from build123d import *

# Parameters (mm, degrees)
BOSS_EXTRUDE1_DEPTH            = 29
SKETCH2_R                      = 2.6
SKETCH2_R_2                    = 1.55
BOSS_EXTRUDE3_DEPTH            = 5
CUT_EXTRUDE1_REACH             = 90.599
CUT_EXTRUDE1_DIRECTION_2_DEPTH = 89.598840586
CUT_EXTRUDE2_REACH             = 90.599
CUT_EXTRUDE2_DIRECTION_2_DEPTH = 89.598840586
FILLET1_R                      = 2
SKETCH6_R                      = 2.6
BOSS_EXTRUDE4_DEPTH            = 1


with BuildPart() as part:
    # Sketch1 → Boss-Extrude1 (new body)
    with BuildSketch(Plane(origin=(0, 0, 0), x_dir=(1, 0, 0), z_dir=(0, 1, 0))):
        Polygon((-13.5, 0), (0, 74.39897269), (13.5, 0), (14.483932895, 0.178538676), (0, 80), (-14.483932895, 0.178538676), align=None)
    extrude(amount=BOSS_EXTRUDE1_DEPTH)

    # Sketch2 → Boss-Extrude3 (add)
    # profile 1 of 8: a face of its own
    with BuildSketch(Plane(origin=(0, 0, 0), x_dir=(1, 0, 0), z_dir=(0, 1, 0))):
        with Locations((11.925707369, -0.285661882)):
            Circle(SKETCH2_R)
        with Locations(Location((11.925707369, -0.285661882, 0), (0, 0, 270))):
            Circle(SKETCH2_R_2, mode=Mode.SUBTRACT)
    # profile 2 of 8: a face of its own
    with BuildSketch(Plane(origin=(0, 0, 0), x_dir=(1, 0, 0), z_dir=(0, 1, 0))):
        with Locations((9.426165905, 13.489398644)):
            Circle(SKETCH2_R)
        with Locations(Location((9.426165905, 13.489398644, 0), (0, 0, 270))):
            Circle(SKETCH2_R_2, mode=Mode.SUBTRACT)
    # profile 3 of 8: a face of its own
    with BuildSketch(Plane(origin=(0, 0, 0), x_dir=(1, 0, 0), z_dir=(0, 1, 0))):
        with Locations((6.926624441, 27.264459169)):
            Circle(SKETCH2_R)
        with Locations(Location((6.926624441, 27.264459169, 0), (0, 0, 270))):
            Circle(SKETCH2_R_2, mode=Mode.SUBTRACT)
    # profile 4 of 8: a face of its own
    with BuildSketch(Plane(origin=(0, 0, 0), x_dir=(1, 0, 0), z_dir=(0, 1, 0))):
        with Locations((4.427082978, 41.039519694)):
            Circle(SKETCH2_R)
        with Locations(Location((4.427082978, 41.039519694, 0), (0, 0, 270))):
            Circle(SKETCH2_R_2, mode=Mode.SUBTRACT)
    # profile 5 of 8: a face of its own
    with BuildSketch(Plane(origin=(0, 0, 0), x_dir=(1, 0, 0), z_dir=(0, 1, 0))):
        with Locations((-11.925707369, -0.285661882)):
            Circle(SKETCH2_R)
        with Locations(Location((-11.925707369, -0.285661882, 0), (0, 0, 90))):
            Circle(SKETCH2_R_2, mode=Mode.SUBTRACT)
    # profile 6 of 8: a face of its own
    with BuildSketch(Plane(origin=(0, 0, 0), x_dir=(1, 0, 0), z_dir=(0, 1, 0))):
        with Locations((-9.426165905, 13.489398644)):
            Circle(SKETCH2_R)
        with Locations(Location((-9.426165905, 13.489398644, 0), (0, 0, 90))):
            Circle(SKETCH2_R_2, mode=Mode.SUBTRACT)
    # profile 7 of 8: a face of its own
    with BuildSketch(Plane(origin=(0, 0, 0), x_dir=(1, 0, 0), z_dir=(0, 1, 0))):
        with Locations((-6.926624441, 27.264459169)):
            Circle(SKETCH2_R)
        with Locations(Location((-6.926624441, 27.264459169, 0), (0, 0, 90))):
            Circle(SKETCH2_R_2, mode=Mode.SUBTRACT)
    # profile 8 of 8: a face of its own
    with BuildSketch(Plane(origin=(0, 0, 0), x_dir=(1, 0, 0), z_dir=(0, 1, 0))):
        with Locations((-4.427082978, 41.039519694)):
            Circle(SKETCH2_R)
        with Locations(Location((-4.427082978, 41.039519694, 0), (0, 0, 90))):
            Circle(SKETCH2_R_2, mode=Mode.SUBTRACT)
    boss_extrude3 = extrude(amount=BOSS_EXTRUDE3_DEPTH)

    # Cut-Extrude1: up to this face of the body (flat: up to its plane)
    cut_extrude1_end = Plane(part.part.faces().sort_by_distance((-6.66752213, 14.905805763, -37.654024776))[0])
    # Sketch4 → Cut-Extrude1 (cut, up to the picked face)
    with BuildSketch(Plane(origin=(0.430326794, 0, 2.371546029), x_dir=(0.9839328946538309, 0, -0.17853867597283662), z_dir=(0.17853867597283662, 0, 0.9839328946538309)), mode=Mode.PRIVATE) as cut_extrude1_sk1:
        Polygon((13.283094078, 5), (9.083094078, 5), (9.083094078, 1.475781549), align=None)
    cut_extrude1_tool1 = split(extrude(cut_extrude1_sk1.sketch, amount=-CUT_EXTRUDE1_REACH, mode=Mode.PRIVATE), bisect_by=cut_extrude1_end, keep=Keep.BOTH, mode=Mode.PRIVATE)
    cut_extrude1 = cut_extrude1_tool1.solids().sort_by(Axis((10.744988, 3.825261, 0.499908), (-0.17853867597283662, 0, -0.9839328946538309)))[0]
    add(cut_extrude1, mode=Mode.SUBTRACT)

    # Sketch4 → Cut-Extrude1 direction 2 (cut)
    with BuildSketch(Plane(origin=(0.430326794, 0, 2.371546029), x_dir=(0.9839328946538309, 0, -0.17853867597283662), z_dir=(0.17853867597283662, 0, 0.9839328946538309))):
        Polygon((13.283094078, 5), (9.083094078, 5), (9.083094078, 1.475781549), align=None)
    cut_extrude1_direction_2 = extrude(amount=CUT_EXTRUDE1_DIRECTION_2_DEPTH, mode=Mode.SUBTRACT)

    # Cut-Extrude2: up to this face of the body (flat: up to its plane)
    cut_extrude2_end = Plane(part.part.faces().sort_by_distance((6.66752213, 14.905805763, -37.654024776))[0])
    # Sketch5 → Cut-Extrude2 (cut, up to the picked face)
    with BuildSketch(Plane(origin=(-0.430326794, 0, 2.371546029), x_dir=(0.9839328946538308, 0, 0.17853867597283732), z_dir=(-0.17853867597283732, 0, 0.9839328946538308)), mode=Mode.PRIVATE) as cut_extrude2_sk1:
        Polygon((-9.083094078, 5), (-9.083094078, 1.475781549), (-13.283094078, 5), align=None)
    cut_extrude2_tool1 = split(extrude(cut_extrude2_sk1.sketch, amount=-CUT_EXTRUDE2_REACH, mode=Mode.PRIVATE), bisect_by=cut_extrude2_end, keep=Keep.BOTH, mode=Mode.PRIVATE)
    cut_extrude2 = cut_extrude2_tool1.solids().sort_by(Axis((-10.744988, 3.825261, 0.499908), (0.17853867597283732, 0, -0.9839328946538308)))[0]
    add(cut_extrude2, mode=Mode.SUBTRACT)

    # Sketch5 → Cut-Extrude2 direction 2 (cut)
    with BuildSketch(Plane(origin=(-0.430326794, 0, 2.371546029), x_dir=(0.9839328946538308, 0, 0.17853867597283732), z_dir=(-0.17853867597283732, 0, 0.9839328946538308))):
        Polygon((-9.083094078, 5), (-9.083094078, 1.475781549), (-13.283094078, 5), align=None)
    cut_extrude2_direction_2 = extrude(amount=CUT_EXTRUDE2_DIRECTION_2_DEPTH, mode=Mode.SUBTRACT)

    # Mirror2: Boss-Extrude3, Cut-Extrude1, Cut-Extrude1 direction 2, Cut-Extrude2, Cut-Extrude2 direction 2 across plane
    add(boss_extrude3.mirror(Plane.ZX.offset(14.5)))
    add(cut_extrude1.mirror(Plane.ZX.offset(14.5)), mode=Mode.SUBTRACT)
    add(cut_extrude1_direction_2.mirror(Plane.ZX.offset(14.5)), mode=Mode.SUBTRACT)
    add(cut_extrude2.mirror(Plane.ZX.offset(14.5)), mode=Mode.SUBTRACT)
    add(cut_extrude2_direction_2.mirror(Plane.ZX.offset(14.5)), mode=Mode.SUBTRACT)

    # Fillet1
    # the kernel refuses this fillet: 2 mm, written as the material it adds along each edge
    with BuildSketch(Plane(origin=(13.5, 5, 0), x_dir=(0, 1, 0), z_dir=(0.9839328946538308, 0, -0.17853867597283668))) as fillet1_piece_1_section:
        with BuildLine():
            CenterArc((FILLET1_R, FILLET1_R), FILLET1_R, 180, 90)
            Line((0, FILLET1_R), (0, 0))
            Line((0, 0), (FILLET1_R, 0))
        make_face()
    fillet1_piece_1 = extrude(amount=6, mode=Mode.PRIVATE)
    fillet1_piece_1 = fillet1_piece_1 & Plane(origin=(11.925707369, 5.699977743, 0.285661882), x_dir=(1, 0, 0), z_dir=(0, -1, 0)) * Cylinder(2.6, 20, mode=Mode.PRIVATE)
    add(fillet1_piece_1)
    with BuildSketch(Plane(origin=(13.5, 24, 0), x_dir=(0, -1, 0), z_dir=(0.9839328946538308, 0, -0.17853867597283668))) as fillet1_piece_2_section:
        with BuildLine():
            CenterArc((FILLET1_R, -FILLET1_R), FILLET1_R, 90, 90)
            Line((0, -FILLET1_R), (0, 0))
            Line((0, 0), (FILLET1_R, 0))
        make_face()
    fillet1_piece_2 = extrude(amount=6, mode=Mode.PRIVATE)
    fillet1_piece_2 = fillet1_piece_2 & Plane(origin=(11.925707369, 23.300022258, 0.285661882), x_dir=(1, 0, 0), z_dir=(0, 1, 0)) * Cylinder(2.6, 20, mode=Mode.PRIVATE)
    add(fillet1_piece_2)
    with BuildSketch(Plane(origin=(-19.403597368, 24, -1.071232056), x_dir=(0, -1, 0), z_dir=(0.9839328946538307, 0, 0.17853867597283735))) as fillet1_piece_3_section:
        with BuildLine():
            CenterArc((FILLET1_R, -FILLET1_R), FILLET1_R, 90, 90)
            Line((0, -FILLET1_R), (0, 0))
            Line((0, 0), (FILLET1_R, 0))
        make_face()
    fillet1_piece_3 = extrude(amount=6, mode=Mode.PRIVATE)
    fillet1_piece_3 = fillet1_piece_3 & Plane(origin=(-11.925707369, 23.777637105, 0.285661882), x_dir=(1, 0, 0), z_dir=(0, 1, 0)) * Cylinder(2.6, 21, mode=Mode.PRIVATE)
    add(fillet1_piece_3)
    with BuildSketch(Plane(origin=(-19.403597368, 5, -1.071232056), x_dir=(-0.17853867597283735, 0, 0.9839328946538307), z_dir=(0.9839328946538307, 0, 0.17853867597283735))) as fillet1_piece_4_section:
        with BuildLine():
            CenterArc((FILLET1_R, -FILLET1_R), FILLET1_R, 90, 90)
            Line((0, -FILLET1_R), (0, 0))
            Line((0, 0), (FILLET1_R, 0))
        make_face()
    fillet1_piece_4 = extrude(amount=6, mode=Mode.PRIVATE)
    fillet1_piece_4 = fillet1_piece_4 & Plane(origin=(-11.925707369, 5.222362792, 0.285661882), x_dir=(1, 0, 0), z_dir=(0, -1, 0)) * Cylinder(2.6, 21, mode=Mode.PRIVATE)
    add(fillet1_piece_4)

    # Sketch6 → Boss-Extrude4 (add)
    with BuildSketch(Plane.XZ):
        with Locations((4.427082978, -41.039519694)):
            Circle(SKETCH6_R)
        with Locations((-4.427082978, -41.039519694)):
            Circle(SKETCH6_R)
        with Locations((-6.926624441, -27.264459169)):
            Circle(SKETCH6_R)
        with Locations((11.925707369, 0.285661882)):
            Circle(SKETCH6_R)
        with Locations((6.926624441, -27.264459169)):
            Circle(SKETCH6_R)
        with Locations((9.426165905, -13.489398644)):
            Circle(SKETCH6_R)
        with Locations((-9.426165905, -13.489398644)):
            Circle(SKETCH6_R)
        with Locations((-11.925707369, 0.285661882)):
            Circle(SKETCH6_R)
    extrude(amount=-BOSS_EXTRUDE4_DEPTH)


solid = part.part
For this review, take the finished solid that the model builds, in its own axes (mm). A direction names the side the tool comes from. Round coordinates to 2 decimals unless told otherwise and drop trailing zeros. Write each loop counter-clockwise with the first axis right and the second up, starting at its lowest first coordinate (ties: lowest second). Pieces come first, ordered by that corner, then holes. Notation, with made-up numbers: (34.5, -27) - (39.5, -27) arc R23 ccw to (39.5, 5) - close; hole circle Ø6 at (25.25, 9.5). An arc over 180 degrees is marked (long way). Write item = value, one per line. Start each with the question number.
1. For faces 1 (the face through (-5.29, 26.57, -28.1)), 2 (the face through (5.964, 2.513, -41.241)), 3 (the face through (-7.026, 14.297, -35.681)), list the 3-axis set-ups (+Z, -Z, +X, -X, +Y, -Y) from which the entire face can be reached by the end or side of a thin tool; tool diameter is ignored.
2. Consider section B-B on y = 14.25. State the section outline as (x, z) points.
3. Consider section C-C on x = -1. State the section outline as (y, z) points.
4. Consider section A-A on z = -22. State the section outline as (x, y) points.
5. Wall thickness on L1, parallel to X at y = 1.5, z = -25; L2, parallel to X at y = 8.25, z = -2; L3, parallel to Y at x = 9, z = -13: over which ranges is each line inside the solid? List them lowest first.
6. For pin 1 Ø2 at (y, z) = (12, -48.5) entering from +X; pin 2 Ø2 at (y, z) = (11.5, -33) entering from +X; pin 3 Ø2.5 at (x, z) = (4.43, -41.04) entering from +Y, all flat-tipped, find the tip position at first contact; note any pin that passes through.
7. Draft analysis for pull direction X (two halves, no side actions). For faces 4 (the face through (-8.463, 2.521, -27.063)), 5 (the face through (4, 1, -41)), 6 (the face through (-14.061, 23.129, 0.253)), 7 (the face through (7.343, 14.297, -39.531)), state which applies: released by +X, released by -X, zero draft, split by the parting line, or undercut.
Evaluation:
q1.face_1 = +Z
q1.face_2 = +Y
q1.face_3 = none
q2.outline = (-14.48, -0.18) - (0, -80) - (14.48, -0.18) - (13.5, 0) - (0, -74.4) - (-13.5, 0) - close
q3.outline = (0, -74.49) - (29, -74.49) - (29, -68.89) - (0, -68.89) - close
q4.outline = (-10.52, 0) - (-9.51, 0) - (-9.51, 29) - (-10.52, 29) - close; (9.51, 0) - (10.52, 0) - (10.52, 29) - (9.51, 29) - close
q5.L1 = -9.98 to -8.96, -8.2 to -5.65, 5.65 to 8.2, 8.96 to 9.98
q5.L2 = -14.15 to -13.14, 13.14 to 14.15
q5.L3 = 0 to 1
q6.pin_1 = 5.9
q6.pin_2 = 8.71
q6.pin_3 = 1
q7.face_4 = undercut
q7.face_5 = undercut
q7.face_6 = released by -X
q7.face_7 = released by +X
